Input: part model. Units: mm. Frame: model coordinates. A direction names the side the tool comes from. Give positions to 0.01 mm unless a question says otherwise; leave off trailing zeros. Write each loop counter-clockwise with the first axis right and the second up, starting at its lowest first coordinate (ties: lowest second). Pieces come first, ordered by that corner, then holes. Notation, with made-up numbers: (3.25, 44) -> (26.25, 44) arc R21 cw to (26.25, 57) -> close; hole circle Ø5 at (57, -19). An arc over 180 degrees is marked (long way). Answer as a JSON object with one key per item and string values. Group by question number.
from build123d import *

# Parameters (mm, degrees)
MODEL_R                 = 16.5
MODEL_R_2               = 0.95
MODEL_R_3               = 1.5
SALIENTE_EXTRUIR3_DEPTH = 3
CROQUIS3_W              = 6.5
CROQUIS3_H              = 6.5
CORTAR_EXTRUIR1_DEPTH   = 2
CROQUIS4_W              = 6.500000001
CROQUIS4_H              = 6.5
CORTAR_EXTRUIR2_DEPTH   = 2


with BuildPart() as part:
    # Model → Saliente-Extruir3 (new body)
    with BuildSketch(Plane.XY):
        with Locations((215.747807914, 241.952019993)):
            Circle(MODEL_R)
        with Locations((215.747807914, 241.952019993)):
            Circle(MODEL_R_2, mode=Mode.SUBTRACT)
        with Locations((215.747807914, 250.952019993)):
            Circle(MODEL_R_3, mode=Mode.SUBTRACT)
        with Locations((215.747807914, 232.952019993)):
            Circle(MODEL_R_3, mode=Mode.SUBTRACT)
        with BuildLine():
            Line((223.122807913, 245.202019993), (221.372807913, 245.202019993))
            ThreePointArc((221.372807913, 245.202019993), (220.842477828, 244.982350079), (220.622807913, 244.452019993))
            Line((220.622807913, 244.452019993), (220.622807913, 239.452019993))
            ThreePointArc((220.622807913, 239.452019993), (220.842477828, 238.921689907), (221.372807913, 238.702019993))
            Line((221.372807913, 238.702019993), (223.122807913, 238.702019993))
            ThreePointArc((223.122807913, 238.702019993), (223.653137999, 238.921689907), (223.872807913, 239.452019993))
            Line((223.872807913, 239.452019993), (223.872807913, 244.452019993))
            ThreePointArc((223.872807913, 244.452019993), (223.653137999, 244.982350079), (223.122807913, 245.202019993))
        make_face(mode=Mode.SUBTRACT)
        with BuildLine():
            Line((208.372807913, 245.202019993), (210.122807913, 245.202019993))
            ThreePointArc((210.122807913, 245.202019993), (210.653137999, 244.982350079), (210.872807913, 244.452019993))
            Line((210.872807913, 244.452019993), (210.872807913, 239.452019993))
            ThreePointArc((210.872807913, 239.452019993), (210.653137999, 238.921689907), (210.122807913, 238.702019993))
            Line((210.122807913, 238.702019993), (208.372807913, 238.702019993))
            ThreePointArc((208.372807913, 238.702019993), (207.842477828, 238.921689907), (207.622807913, 239.452019993))
            Line((207.622807913, 239.452019993), (207.622807913, 244.452019993))
            ThreePointArc((207.622807913, 244.452019993), (207.842477828, 244.982350079), (208.372807913, 245.202019993))
        make_face(mode=Mode.SUBTRACT)
    extrude(amount=SALIENTE_EXTRUIR3_DEPTH)

    # Croquis3 → Cortar-Extruir1 (cut)
    with BuildSketch(Plane.XY.offset(3)):
        with Locations((215.747807914, 250.952019993)):
            Rectangle(CROQUIS3_W, CROQUIS3_H)
    extrude(amount=-CORTAR_EXTRUIR1_DEPTH, mode=Mode.SUBTRACT)

    # Croquis4 → Cortar-Extruir2 (cut)
    with BuildSketch(Plane.XY.offset(3)):
        with Locations((215.747807914, 232.952019993)):
            Rectangle(CROQUIS4_W, CROQUIS4_H)
    extrude(amount=-CORTAR_EXTRUIR2_DEPTH, mode=Mode.SUBTRACT)


solid = part.part
1. Section A-A (y = 240). Return the cut outline in (x, z).
2. Reachability of faces 5 (the face through (210.873, 242, 1)), 6 (the face through (216, 229.702, 2)), 7 (the face through (216, 239, 0)) from +Z, -Z, +X, -X, +Y, -Y: full face, straight path, thin tool, end or side. Return the list, or none.
3. Section C-C (z = 2). Return the cut outline in (x, y).
4. Section B-B (x = 216). Return the cut outline in (y, z), plus the area to 3 significant figures.
5. Line query: line 1 (X direction, y = 242.5, z = 0.6); line 2 (X direction, y = 239.5, z = 0.25); line 3 (Y direction, x = 223, z = 2.95). Output: solid intervals per line, ascending.
6. Contact query for flat-ended pins moving along their axis: pin 1 Ø1.5 at (y, z) = (241, 2) entering from +X; pin 2 Ø0.6 at (x, z) = (214.5, 2.5) entering from -Y; pin 3 Ø1 at (x, z) = (217, 2.5) entering from +Y; pin 4 Ø1.1 at (x, y) = (215.75, 241.95) entering from +Z. Output: stop coordinate, or through.
7. Section D-D (y = 235.5). Return the cut outline in (x, z).
8. Mould query, pull axis X, two halves, no side actions, for faces 1 (the face through (216, 239, 3)), 2 (the face through (213.6, 258.31, 1.48)), 3 (the face through (212.498, 251, 2)), 4 (the face through (216, 247.702, 2)). Classes: pulls with the +X half, pulls with the -X half, needs draft (parallel to the pull), parting line crosses it, or undercut.
Working result:
{
 "1": {"outline": "(199.36, 0) -> (207.62, 0) -> (207.62, 3) -> (199.36, 3) -> close; (210.87, 0) -> (220.62, 0) -> (220.62, 3) -> (210.87, 3) -> close; (223.87, 0) -> (232.13, 0) -> (232.13, 3) -> (223.87, 3) -> close"},
 "2": {"face 5": "+Z, -Z", "face 6": "+Z", "face 7": "-Z, +X, -X, +Y, -Y"},
 "3": {"outline": "circle Ø33 at (215.75, 241.95); hole (207.62, 239.45) arc R0.75 ccw to (208.37, 238.7) -> (210.12, 238.7) arc R0.75 ccw to (210.87, 239.45) -> (210.87, 244.45) arc R0.75 ccw to (210.12, 245.2) -> (208.37, 245.2) arc R0.75 ccw to (207.62, 244.45) -> close; hole (212.5, 229.7) -> (219, 229.7) -> (219, 236.2) -> (212.5, 236.2) -> close; hole (212.5, 247.7) -> (219, 247.7) -> (219, 254.2) -> (212.5, 254.2) -> close; hole circle Ø1.9 at (215.75, 241.95); hole (220.62, 239.45) arc R0.75 ccw to (221.37, 238.7) -> (223.12, 238.7) arc R0.75 ccw to (223.87, 239.45) -> (223.87, 244.45) arc R0.75 ccw to (223.12, 245.2) -> (221.37, 245.2) arc R0.75 ccw to (220.62, 244.45) -> close"},
 "4": {"outline": "(225.45, 0) -> (231.47, 0) -> (231.47, 1) -> (229.7, 1) -> (229.7, 3) -> (225.45, 3) -> close; (234.43, 0) -> (241.04, 0) -> (241.04, 3) -> (236.2, 3) -> (236.2, 1) -> (234.43, 1) -> close; (242.87, 0) -> (249.47, 0) -> (249.47, 1) -> (247.7, 1) -> (247.7, 3) -> (242.87, 3) -> close; (252.43, 0) -> (258.45, 0) -> (258.45, 3) -> (254.2, 3) -> (254.2, 1) -> (252.43, 1) -> close", "area": "61.6 mm^2"},
 "5": {"line 1": "x = 199.26 to 207.62, 210.87 to 214.97, 216.52 to 220.62, 223.87 to 232.24", "line 2": "x = 199.43 to 207.62, 210.87 to 220.62, 223.87 to 232.06", "line 3": "y = 227.13 to 238.7, 245.2 to 256.77"},
 "6": {"pin 1": "stops at x = 232.25", "pin 2": "stops at y = 225.48", "pin 3": "stops at y = 258.43", "pin 4": "passes through"},
 "7": {"outline": "(200.56, 0) -> (230.93, 0) -> (230.93, 3) -> (219, 3) -> (219, 1) -> (212.5, 1) -> (212.5, 3) -> (200.56, 3) -> close"},
 "8": {"face 1": "needs draft", "face 2": "parting line crosses it", "face 3": "undercut", "face 4": "undercut"}
}
